Work out the finished part from the listing and answer in its coordinate system (mm). Face numbers are marked on the shaded views. A direction names the side the tool comes from. Coordinates: 2 decimals unless noted, no trailing zeros. Order: outer loops, then holes, each group sorted by start corner. A loop starts at its lowest first (then second) coordinate and runs counter-clockwise, first axis right, second up. Notation, with made-up numbers: (8.5, 52) -> (55.5, 52) arc R14 cw to (55.5, 58) -> close; hole circle Ø11 at (84, 75.5). An arc over 180 degrees is marked (long way). Use one line per item in the form item = value.
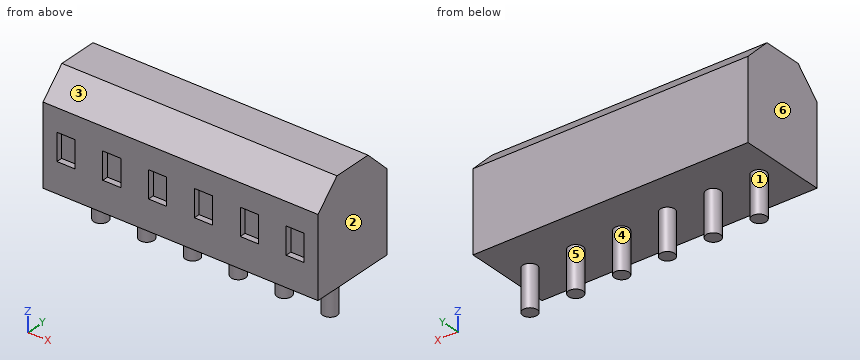
from build123d import *

# Parameters (mm, degrees)
SKETCH_1_W                 = 22.86
SKETCH_1_H                 = 7.3
EXTRUDE_1_DEPTH            = 8.6
CHAMFER_1_SIZE             = 2
SKETCH_2_W                 = 1.5
SKETCH_2_H                 = 2.244760595
CUT_EXTRUDE_1_DEPTH        = 0.5
PATTERN_LINEAR_1_COUNT     = 3
PATTERN_LINEAR_1_PITCH     = 3.81
PATTERN_LINEAR_1_COL_COUNT = 4
PATTERN_LINEAR_1_COL_PITCH = 3.81
SKETCH_3_R                 = 0.6
EXTRUDE_2_DEPTH            = 3.4
PATTERN_LINEAR_2_COUNT     = 4
PATTERN_LINEAR_2_PITCH     = 3.81
PATTERN_LINEAR_2_COL_COUNT = 3
PATTERN_LINEAR_2_COL_PITCH = 3.81
PATTERN_LINEAR_3_COUNT     = 2
PATTERN_LINEAR_3_PITCH     = 3.81


with BuildPart() as part:
    # 草图1 → 凸台-拉伸1 (new body)
    with BuildSketch(Plane.XY):
        with Locations((11.43, 3.65)):
            Rectangle(SKETCH_1_W, SKETCH_1_H)
    extrude(amount=EXTRUDE_1_DEPTH)

    # 倒角1
    chamfer_1_edges = [part.edges().sort_by_distance(p)[0] for p in [
        (11.43, 7.3, 8.6),
        (11.43, 0, 8.6),
    ]]
    chamfer(chamfer_1_edges, length=CHAMFER_1_SIZE)

    # 草图2 → 切除-拉伸1 (cut)
    with BuildSketch(Plane.XZ):
        with Locations((13.335, 3.602057757)):
            Rectangle(SKETCH_2_W, SKETCH_2_H)
    cut_extrude_1 = extrude(amount=-CUT_EXTRUDE_1_DEPTH, mode=Mode.SUBTRACT)

    # 阵列(线性)1: 切除-拉伸1 ×3
    with Locations(*[(i * PATTERN_LINEAR_1_PITCH, 0, 0) for i in range(1, PATTERN_LINEAR_1_COUNT)]):
        add(cut_extrude_1, mode=Mode.SUBTRACT)

    # 阵列(线性)1 col: 切除-拉伸1 ×4
    with Locations(*[(-i * PATTERN_LINEAR_1_COL_PITCH, 0, 0) for i in range(1, PATTERN_LINEAR_1_COL_COUNT)]):
        add(cut_extrude_1, mode=Mode.SUBTRACT)

    # 草图3 → 凸台-拉伸2 (add)
    with BuildSketch(Plane(origin=(0, 0, 0), x_dir=(-1, 0, 0), z_dir=(0, 0, -1))):
        with Locations((-13.335, 3.7)):
            Circle(SKETCH_3_R)
    extrude_2 = extrude(amount=EXTRUDE_2_DEPTH)

    # 阵列(线性)2: 凸台-拉伸2 ×4
    with Locations(*[(-i * PATTERN_LINEAR_2_PITCH, 0, 0) for i in range(1, PATTERN_LINEAR_2_COUNT)]):
        add(extrude_2)

    # 阵列(线性)2 col: 凸台-拉伸2 ×3
    with Locations(*[(i * PATTERN_LINEAR_2_COL_PITCH, 0, 0) for i in range(1, PATTERN_LINEAR_2_COL_COUNT)]):
        add(extrude_2)

    # 阵列(线性)3: 凸台-拉伸2 ×2
    with Locations(*[(-i * PATTERN_LINEAR_3_PITCH, 0, 0) for i in range(1, PATTERN_LINEAR_3_COUNT)]):
        add(extrude_2)


solid = part.part
(1) Section A-A on z = 3.25 is taken. Write down the section's boundary in (x, y) (3 decimals).
Data:
outline = (0, 0) -> (1.155, 0) -> (1.155, 0.5) -> (2.655, 0.5) -> (2.655, 0) -> (4.965, 0) -> (4.965, 0.5) -> (6.465, 0.5) -> (6.465, 0) -> (8.775, 0) -> (8.775, 0.5) -> (10.275, 0.5) -> (10.275, 0) -> (12.585, 0) -> (12.585, 0.5) -> (14.085, 0.5) -> (14.085, 0) -> (16.395, 0) -> (16.395, 0.5) -> (17.895, 0.5) -> (17.895, 0) -> (20.205, 0) -> (20.205, 0.5) -> (21.705, 0.5) -> (21.705, 0) -> (22.86, 0) -> (22.86, 7.3) -> (0, 7.3) -> close
(2) Section D-D on z = 7.75 is taken. Write down the section's boundary in (x, y), plus the area to 3 significant figures.
Data:
outline = (0, 1.15) -> (22.86, 1.15) -> (22.86, 6.15) -> (0, 6.15) -> close
area = 114 mm²
(3) Section C-C on x = 18.25 is taken. Write down the section's boundary in (y, z).
Data:
outline = (0, 0) -> (7.3, 0) -> (7.3, 6.6) -> (5.3, 8.6) -> (2, 8.6) -> (0, 6.6) -> close
(4) Straight lines are drawn through the part: line 1 along Y through (x, z) = (1.5, 3.5); line 2 along Z through (x, y) = (11.75, 4.75); line 3 along X through (y, z) = (3.5, -1.25). For each, find the intervals that lie inside material, in ascending order.
Data:
line_1 = 0.5 to 7.3
line_2 = 0 to 8.6
line_3 = 1.34 to 2.47, 5.15 to 6.28, 8.96 to 10.09, 12.77 to 13.9, 16.58 to 17.71, 20.39 to 21.52
(5) Each of these flat-tipped pins is pushed along its axis until it touches: P1, Ø0.8, axis at x = 13.5, z = 4, coming from the -Y side; P2, Ø1, axis at x = 8, y = 4, coming from the -Z side. Where does it stop, or does it pass through?
Data:
P1 = 0.5
P2 = 0
(6) Section B-B on y = 3.7 is taken. Write down the section's boundary in (x, z) (3 decimals), plus the area to 3 significant figures.
Data:
outline = (0, 0) -> (1.305, 0) -> (1.305, -3.4) -> (2.505, -3.4) -> (2.505, 0) -> (5.115, 0) -> (5.115, -3.4) -> (6.315, -3.4) -> (6.315, 0) -> (8.925, 0) -> (8.925, -3.4) -> (10.125, -3.4) -> (10.125, 0) -> (12.735, 0) -> (12.735, -3.4) -> (13.935, -3.4) -> (13.935, 0) -> (16.545, 0) -> (16.545, -3.4) -> (17.745, -3.4) -> (17.745, 0) -> (20.355, 0) -> (20.355, -3.4) -> (21.555, -3.4) -> (21.555, 0) -> (22.86, 0) -> (22.86, 8.6) -> (0, 8.6) -> close
area = 221 mm²
(7) Which of the six approach directions +Z, -Z, +X, -X, +Y, -Y give full straight-line access (tool end or side, diameter ignored) to the marked faces 5 and 6?
Data:
face_5 = -Z
face_6 = +Z, -Z, -X, +Y, -Y
(8) The mould has two halves that part along X. Classify the marked faces 1, 2, 3 and 4: released by +X, released by -X, zero draft, split by the parting line, or undercut.
Data:
face_1 = undercut
face_2 = released by +X
face_3 = zero draft
face_4 = undercut
